Model file for the job. Use its own axes, mm. Face numbers are marked on the shaded views. A direction names the side the tool comes from. Coordinates: 2 decimals unless noted, no trailing zeros. Loops run counter-clockwise (first coordinate to the right, second up) from the corner with the lowest first, then second, coordinate; pieces in that order, holes last. Notation, with made-up numbers: (-14, 12.25) -> (32, 12.25) arc R19 cw to (32, 48.25) -> close; hole circle Ø1 at (-22.5, -12). An arc over 180 degrees is marked (long way). Use one line per item in the form item = value.
```python
from build123d import *

# Parameters (mm, degrees)
SKETCH2_R               = 3.5
BOSS_EXTRUDE1_DEPTH     = 34
SKETCH19_R              = 8.25
SKETCH19_R_2            = 3.5
BOSS_EXTRUDE3_DEPTH     = 3.5
BOSS_EXTRUDE2_DEPTH     = 3.5
SKETCH4_R               = 10
CUT_EXTRUDE1_DEPTH      = 3.5
LPATTERN4_COUNT         = 2
LPATTERN4_PITCH         = 34.5
CUT_EXTRUDE3_DEPTH      = 48.681233293
SKETCH7_R               = 13.5
CUT_EXTRUDE4_DEPTH      = 4.5
LPATTERN3_COUNT         = 2
LPATTERN3_PITCH         = 26.5
M2_TAPPED_HOLE1_D       = 1.6
M2_TAPPED_HOLE1_DEPTH   = 5.5
M2_TAPPED_HOLE1_TIP     = 0.480688495
SKETCH17_R              = 2
CUT_EXTRUDE5_DEPTH      = 8
CUT_EXTRUDE6_REACH      = 50.532
CUT_EXTRUDE6_END_RADIUS = 19
SKETCH20_R              = 9.75
CUT_EXTRUDE7_DEPTH      = 6.25
SKETCH21_R              = 8.5
CUT_EXTRUDE8_DEPTH      = 0.5
SKETCH22_R              = 9.5
CUT_EXTRUDE9_DEPTH      = 5.75
SKETCH23_R              = 10.5
CUT_EXTRUDE10_DEPTH     = 0.5
SKETCH24_R              = 9.5
CUT_EXTRUDE11_DEPTH     = 2


with BuildPart() as part:
    # Sketch2 → Boss-Extrude1 (new body)
    with BuildSketch(Plane(origin=(0, 0, 0), x_dir=(1, 0, 0), z_dir=(0, 1, 0))):
        with BuildLine():
            Line((-3.5, -19), (-3.5, 19))
            Line((-3.5, 19), (0, 19))
            ThreePointArc((0, 19), (19, 0), (0, -19))
            Line((0, -19), (-3.5, -19))
        make_face()
        with Locations(Location((7.75, 0, 0), (0, 0, 270))):
            Circle(SKETCH2_R, mode=Mode.SUBTRACT)
    extrude(amount=BOSS_EXTRUDE1_DEPTH)

    # Sketch19 → Boss-Extrude3 (add)
    with BuildSketch(Plane(origin=(0, 34, 0), x_dir=(1, 0, 0), z_dir=(0, 1, 0))):
        with Locations(Location((7.75, 0, 0), (0, 0, 270))):
            Circle(SKETCH19_R)
        with Locations(Location((7.75, 0, 0), (0, 0, 270))):
            Circle(SKETCH19_R_2, mode=Mode.SUBTRACT)
    extrude(amount=BOSS_EXTRUDE3_DEPTH)

    # Sketch3 → Boss-Extrude2 (add)
    with BuildSketch(Plane.XY.offset(19)):
        with BuildLine():
            Line((-6.75, 0), (-3.5, 0))
            Line((-3.5, 0), (-3.5, 26))
            Line((-3.5, 26), (-6.75, 26))
            ThreePointArc((-6.75, 26), (-19.75, 13), (-6.75, 0))
        make_face()
    boss_extrude2 = extrude(amount=-BOSS_EXTRUDE2_DEPTH)

    # Sketch4 → Cut-Extrude1 (cut)
    with BuildSketch(Plane.XY.offset(19)):
        with Locations(Location((-6.75, 13, 0), (0, 0, 312.454150204))):
            Circle(SKETCH4_R)
    cut_extrude1 = extrude(amount=-CUT_EXTRUDE1_DEPTH, mode=Mode.SUBTRACT)

    # LPattern4: Boss-Extrude2, Cut-Extrude1 ×2
    with Locations(*[(0, 0, -i * LPATTERN4_PITCH) for i in range(1, LPATTERN4_COUNT)]):
        add(boss_extrude2)
        add(cut_extrude1, mode=Mode.SUBTRACT)

    # Sketch6 → Cut-Extrude3 (cut, through all)
    with BuildSketch(Plane(origin=(-3.5, 0, 0), x_dir=(0, 0, -1), z_dir=(1, 0, 0))):
        with BuildLine():
            Line((11, 21.25), (-11, 21.25))
            Line((-11, 21.25), (-11, 9.75))
            ThreePointArc((-11, 9.75), (-10.560660172, 8.689339828), (-9.5, 8.25))
            Line((-9.5, 8.25), (9.5, 8.25))
            ThreePointArc((9.5, 8.25), (10.560660172, 8.689339828), (11, 9.75))
            Line((11, 9.75), (11, 21.25))
        make_face()
    extrude(amount=CUT_EXTRUDE3_DEPTH, mode=Mode.SUBTRACT)

    # Sketch7 → Cut-Extrude4 (cut)
    with BuildSketch(Plane(origin=(0, 0, 15.5), x_dir=(-1, 0, 0), z_dir=(0, 0, -1))):
        with Locations((6.75, 13)):
            Circle(SKETCH7_R)
    cut_extrude4 = extrude(amount=CUT_EXTRUDE4_DEPTH, mode=Mode.SUBTRACT)

    # LPattern3: Cut-Extrude4 ×2
    with Locations(*[(0, 0, -i * LPATTERN3_PITCH) for i in range(1, LPATTERN3_COUNT)]):
        add(cut_extrude4, mode=Mode.SUBTRACT)

    # M2 Tapped Hole1
    with Locations(Plane.ZY.offset(3.5)):
        with Locations((11, 31.5)):
            Hole(M2_TAPPED_HOLE1_D / 2, depth=M2_TAPPED_HOLE1_DEPTH)
            with Locations((0, 0, -(M2_TAPPED_HOLE1_DEPTH + M2_TAPPED_HOLE1_TIP / 2))):  # 118° drill point
                Cone(0, M2_TAPPED_HOLE1_D / 2, M2_TAPPED_HOLE1_TIP, mode=Mode.SUBTRACT)

    # Sketch17 → Cut-Extrude5 (cut)
    with BuildSketch(Plane.ZY.offset(3.5)):
        with Locations((-14.5, 30)):
            Circle(SKETCH17_R)
    extrude(amount=-CUT_EXTRUDE5_DEPTH, mode=Mode.SUBTRACT)

    # Cut-Extrude6: up to this cylinder (the profile starts inside it)
    cut_extrude6_end = Plane(origin=(0, 29.282291, 0), z_dir=(0, -1, 0)) * Cylinder(CUT_EXTRUDE6_END_RADIUS, 140.064, mode=Mode.PRIVATE)
    # Sketch18 → Cut-Extrude6 (cut, up to the surface)
    with BuildSketch(Plane.ZY.offset(-4.5), mode=Mode.PRIVATE) as cut_extrude6_sk1:
        with BuildLine():
            Line((-19, 24.5), (-13.5, 24.5))
            ThreePointArc((-13.5, 24.5), (-12.439339828, 24.939339828), (-12, 26))
            Line((-12, 26), (-12, 34))
            Line((-12, 34), (-19, 34))
            Line((-19, 34), (-19, 24.5))
        make_face()
    cut_extrude6_tool1 = extrude(cut_extrude6_sk1.sketch, amount=-CUT_EXTRUDE6_REACH, mode=Mode.PRIVATE) & cut_extrude6_end
    add(cut_extrude6_tool1.solids().sort_by_distance((4.5, 29.282291, -15.523149))[0], mode=Mode.SUBTRACT)

    # Sketch20 → Cut-Extrude7 (cut)
    with BuildSketch(Plane.XZ.offset(-21.25)):
        with Locations(Location((7.75, 0, 0), (0, 0, 270))):
            Circle(SKETCH20_R)
    extrude(amount=-CUT_EXTRUDE7_DEPTH, mode=Mode.SUBTRACT)

    # Sketch21 → Cut-Extrude8 (cut)
    with BuildSketch(Plane.XZ.offset(-27.5)):
        with Locations(Location((7.75, 0, 0), (0, 0, 270))):
            Circle(SKETCH21_R)
    extrude(amount=-CUT_EXTRUDE8_DEPTH, mode=Mode.SUBTRACT)

    # Sketch22 → Cut-Extrude9 (cut)
    with BuildSketch(Plane(origin=(0, 8.25, 0), x_dir=(1, 0, 0), z_dir=(0, 1, 0))):
        with Locations(Location((7.75, 0, 0), (0, 0, 270))):
            Circle(SKETCH22_R)
    extrude(amount=-CUT_EXTRUDE9_DEPTH, mode=Mode.SUBTRACT)

    # Sketch23 → Cut-Extrude10 (cut)
    with BuildSketch(Plane(origin=(0, 2.5, 0), x_dir=(1, 0, 0), z_dir=(0, 1, 0))):
        with Locations(Location((7.75, 0, 0), (0, 0, 270))):
            Circle(SKETCH23_R)
    extrude(amount=-CUT_EXTRUDE10_DEPTH, mode=Mode.SUBTRACT)

    # Sketch24 → Cut-Extrude11 (cut)
    with BuildSketch(Plane(origin=(0, 2, 0), x_dir=(1, 0, 0), z_dir=(0, 1, 0))):
        with Locations(Location((7.75, 0, 0), (0, 0, 270))):
            Circle(SKETCH24_R)
    extrude(amount=-CUT_EXTRUDE11_DEPTH, mode=Mode.SUBTRACT)


solid = part.part
```
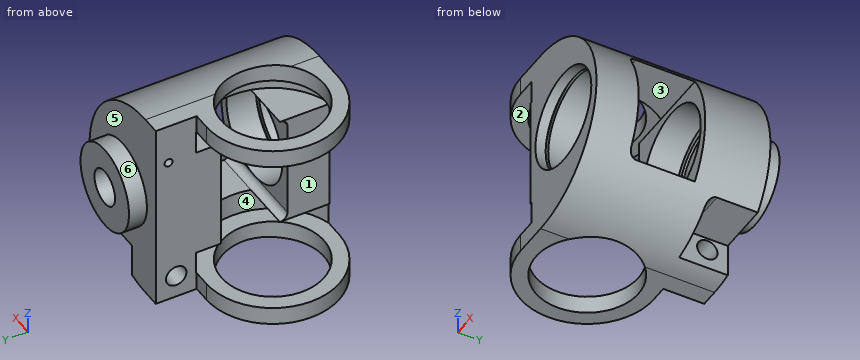
Q1. Band-saw the part on D-D, the plane z = -6. State how many separate pieces and enclosed holes the cut face has, and give its area (3 significant figures).
Result:
separate_pieces = 3
enclosed_holes = 0
area = 267 mm2
Q2. Mould opens along Y. For the marked faces 4, 5 and 6 say: released by +Y, released by -Y, zero draft, split by the parting line, or undercut.
Result:
face_4 = undercut
face_5 = released by +Y
face_6 = zero draft
Q3. Band-saw the part on C-C, the plane y = 9. Write the cut outline in (x, z).
Result:
outline = (-19.12, -19) -> (-15.92, -19) -> (-15.92, -15.5) -> (-19.12, -15.5) -> close; (-19.12, 15.5) -> (-15.92, 15.5) -> (-15.92, 19) -> (-19.12, 19) -> close; (-3.5, -11) -> (6.14, -11) -> (6.14, -15.5) -> (2.42, -15.5) -> (2.42, -18.85) arc R19 ccw to (15.63, -10.8) -> (-3.5, -10.8) -> close; (-3.5, 10.8) -> (15.63, 10.8) arc R19 ccw to (2.42, 18.85) -> (2.42, 15.5) -> (6.14, 15.5) -> (6.14, 11) -> (-3.5, 11) -> close
Q4. Pin check, flat tips, straight feed: pin 1 Ø5 at (x, y) = (4, 6.5) entering from -Z; pin 2 Ø5 at (x, y) = (-6.5, 18.5) entering from +Z; pin 3 Ø1 at (x, z) = (-4.5, -17.5) entering from +Y; pin 4 Ø12 at (x, y) = (8.5, 19) entering from -Z. Stop position of each tip, or through.
Result:
pin_1 = -18.94
pin_2 = through
pin_3 = 26
pin_4 = -18.83
Q5. Which spindle directions (+Z, -Z, +X, -X, +Y, -Y) get a long thin tool onto all of the face, cutting with end or side? Do the marked faces 1, 2 and 3. Say none if no direction does.
Result:
face_1 = -X, +Y, -Y
face_2 = -X
face_3 = +X, -X
Q6. Band-saw the part on B-B, the plane x = -5. Write the cut outline in (y, z), and give its area (3 significant figures).
Result:
outline = (0, -19) -> (3.15, -19) -> (3.15, -15.5) -> (0, -15.5) -> close; (0, 15.5) -> (3.15, 15.5) -> (3.15, 19) -> (0, 19) -> close; (22.85, -19) -> (26, -19) -> (26, -15.5) -> (22.85, -15.5) -> close; (22.85, 15.5) -> (26, 15.5) -> (26, 19) -> (22.85, 19) -> close
area = 44.2 mm2
Q7. Wall check: line 1 along Z through (x, y) = (-3, 24); line 2 along Z through (x, y) = (-16, 17); line 3 along X through (y, z) = (5.1, 0). Give the ranges that are in metal, low to high.
Result:
line_1 = -19 to -15.5, -11 to 11, 15.5 to 19
line_2 = -19 to -15.5, 15.5 to 19
line_3 = -3.5 to -1.75, 17.25 to 19
Q8. Band-saw the part on A-A, the plane y = 30. Write the cut outline in (x, z), and give its area (3 significant figures).
Result:
outline = (-3.5, -19) -> (0, -19) arc R19 ccw to (4.5, -18.46) -> (4.5, -16.5) -> (-3.5, -16.5) -> close; (-3.5, -12.5) -> (4.5, -12.5) -> (4.5, -12) -> (14.73, -12) arc R19 ccw to (0, 19) -> (-3.5, 19) -> close; hole circle Ø7 at (7.75, 0)
area = 589 mm2
